Verification items for the finished model (mm, model axes). A direction names the side the tool comes from. Round coordinates to 2 decimals unless told otherwise and drop trailing zeros. Write each loop counter-clockwise with the first axis right and the second up, starting at its lowest first coordinate (ties: lowest second). Pieces come first, ordered by that corner, then holes. Notation, with made-up numbers: (74.5, -19.75) - (119.5, -19.75) arc R17 cw to (119.5, -13.75) - close; hole circle Ø5 at (68.5, 53). An arc over 180 degrees is marked (long way). Answer as a JSON object with one key per item and string values.
```python
from build123d import *

# Parameters (mm, degrees)
F1_DEPTH = 101.6
F2_DEPTH = 12.7
F3_R     = 22.225
F3_R_2   = 2.55
F4_DEPTH = 12.701
F5_DEPTH = 101.6


with BuildPart() as f1:
    # F0 (on Right) → F1 (new body)
    with BuildSketch(Plane.YZ):
        with BuildLine():
            ThreePointArc((-44.45, -31.75), (-40.730256, -40.730256), (-31.75, -44.45))
            Line((-31.75, -44.45), (-31.75, 38.1))
            Line((-31.75, 38.1), (-31.75, 44.45))
            ThreePointArc((-31.75, 44.45), (-40.730256, 40.730256), (-44.45, 31.75))
            Line((-44.45, 31.75), (-44.45, -31.75))
        make_face()
    extrude(amount=F1_DEPTH)

    # F0 (on Right) → F2 (join)
    with BuildSketch(Plane.YZ):
        with BuildLine():
            Line((-31.75, -44.45), (38.1, -44.45))
            ThreePointArc((38.1, -44.45), (42.590128, -42.590128), (44.45, -38.1))
            Line((44.45, -38.1), (44.45, 38.1))
            Line((44.45, 38.1), (-31.75, 38.1))
            Line((-31.75, 38.1), (-31.75, -44.45))
        make_face()
    extrude(amount=F2_DEPTH)

    # F3 (on face) → F4 (cut, through all)
    with BuildSketch(Plane(origin=(0, -31.75, 0), x_dir=(-1, 0, 0), z_dir=(0, 1, 0))):
        with Locations((-57.15, 0)):
            Circle(F3_R)
        with Locations((-33.65, -23.5)):
            Circle(F3_R_2)
        with Locations((-80.65, -23.5)):
            Circle(F3_R_2)
        with Locations((-80.65, 23.5)):
            Circle(F3_R_2)
        with Locations((-33.65, 23.5)):
            Circle(F3_R_2)
    extrude(amount=-F4_DEPTH, mode=Mode.SUBTRACT)

    # F0 (on Right) → F5 (join)
    with BuildSketch(Plane.YZ):
        with BuildLine():
            Line((-31.75, 44.45), (-31.75, 38.1))
            Line((-31.75, 38.1), (44.45, 38.1))
            ThreePointArc((44.45, 38.1), (42.590128, 42.590128), (38.1, 44.45))
            Line((38.1, 44.45), (-31.75, 44.45))
        make_face()
    extrude(amount=F5_DEPTH)


solid = f1.part
```
1. Material ranges on probe 1 along X at (y, z) = (-34, -23); probe 2 along Z at (x, y) = (33, -41); probe 3 along Z at (x, y) = (55.5, -13), recorded low to high. Write a range as from..to.
Completed:
{"probe 1": "x = 0..31.15, 36.15..78.15, 83.15..101.6", "probe 2": "z = -40.45..-25.97, -21.03..21.03, 25.97..40.45", "probe 3": "z = 38.1..44.45"}
2. Go/stop test with flat-tipped pins: pin 1 (12 mm diameter, centred on y = 26.5, z = -14.5, fed in from +X); pin 2 (8 mm diameter, centred on x = 33.65, z = 23.5, fed in from +Y); pin 3 (4.5 mm diameter, centred on x = 80.65, z = -23.5, fed in from +Y); pin 4 (1.5 mm diameter, centred on x = 58, y = -3.5, fed in from -Z). Record where each tip stops, or that it passes through.
Completed:
{"pin 1": "stops at x = 12.7", "pin 2": "stops at y = -31.75", "pin 3": "passes through", "pin 4": "stops at z = 38.1"}
3. Cross-section at D-D (x = 33.5). Record the boundary of the cut face in (y, z), plus the area to 3 significant figures.
Completed:
{"outline": "(-44.45, -31.75) arc R12.7 ccw to (-31.75, -44.45) - (-31.75, -26.05) - (-44.45, -26.05) - close; (-44.45, -20.95) - (-31.75, -20.95) - (-31.75, 20.95) - (-44.45, 20.95) - close; (-44.45, 26.05) - (-31.75, 26.05) - (-31.75, 38.1) - (44.45, 38.1) arc R6.35 ccw to (38.1, 44.45) - (-31.75, 44.45) arc R12.7 ccw to (-44.45, 31.75) - close", "area": "1,410 mm^2"}
4. Cross-section at B-B (x = 49.5). Record the boundary of the cut face in (y, z), plus the area to 4 significant figures.
Completed:
{"outline": "(-44.45, -31.75) arc R12.7 ccw to (-31.75, -44.45) - (-31.75, -20.87) - (-44.45, -20.87) - close; (-44.45, 20.87) - (-31.75, 20.87) - (-31.75, 38.1) - (44.45, 38.1) arc R6.35 ccw to (38.1, 44.45) - (-31.75, 44.45) arc R12.7 ccw to (-44.45, 31.75) - close", "area": "1,005 mm^2"}
5. Access from +Z, -Z, +X, -X, +Y, -Y to the whole of each face (thin tool, end or side, straight path). Record for faces 5 (the face through (57, 6, 38.1)), 6 (the face through (101.6, -33, 10)).
Completed:
{"face 5": "-Z, +X, +Y", "face 6": "+Z, -Z, +X, +Y, -Y"}
6. Cross-section at A-A (z = 0). Record the boundary of the cut face in (x, y) (3 decimals).
Completed:
{"outline": "(0, -44.45) - (34.925, -44.45) - (34.925, -31.75) - (12.7, -31.75) - (12.7, 44.45) - (0, 44.45) - close; (79.375, -44.45) - (101.6, -44.45) - (101.6, -31.75) - (79.375, -31.75) - close"}
7. Cross-section at C-C (y = -34.5). Record the boundary of the cut face in (x, z) (3 decimals), plus the area to 3 significant figures.
Completed:
{"outline": "(0, -44.149) - (101.6, -44.149) - (101.6, 44.149) - (0, 44.149) - close; hole circle Ø5.1 at (33.65, -23.5); hole circle Ø5.1 at (33.65, 23.5); hole circle Ø44.45 at (57.15, 0); hole circle Ø5.1 at (80.65, -23.5); hole circle Ø5.1 at (80.65, 23.5)", "area": "7,340 mm^2"}
8. Mould release check, pull along Z, two halves, no side actions. Record for faces 1 (the face through (50.09, -40.63, 40.83)), 2 (the face through (6, 3, -44.45)), 3 (the face through (31.22, -38.01, 24.27)), 4 (the face through (6, 44.45, -1)): released by +Z, released by -Z, zero draft, split by the parting line, or undercut.
Completed:
{"face 1": "released by +Z", "face 2": "released by -Z", "face 3": "undercut", "face 4": "zero draft"}
